Source: three-view drawing plus pictorial views. Frame: mm from the lowest corner of the part. A direction names the side the tool comes from. Coordinates: 2 decimals unless noted, no trailing zeros. Order: outer loops, then holes, each group sorted by start corner. A loop starts at its lowest first (then second) coordinate and runs counter-clockwise, first axis right, second up. Notation, with made-up numbers: (37, 81.5) - (67, 81.5) arc R19 cw to (67, 98.5) - close; hole circle Ø8 at (-36.75, 62.5). An arc over 180 degrees is marked (long way). One line per question, with ' | ' between items.
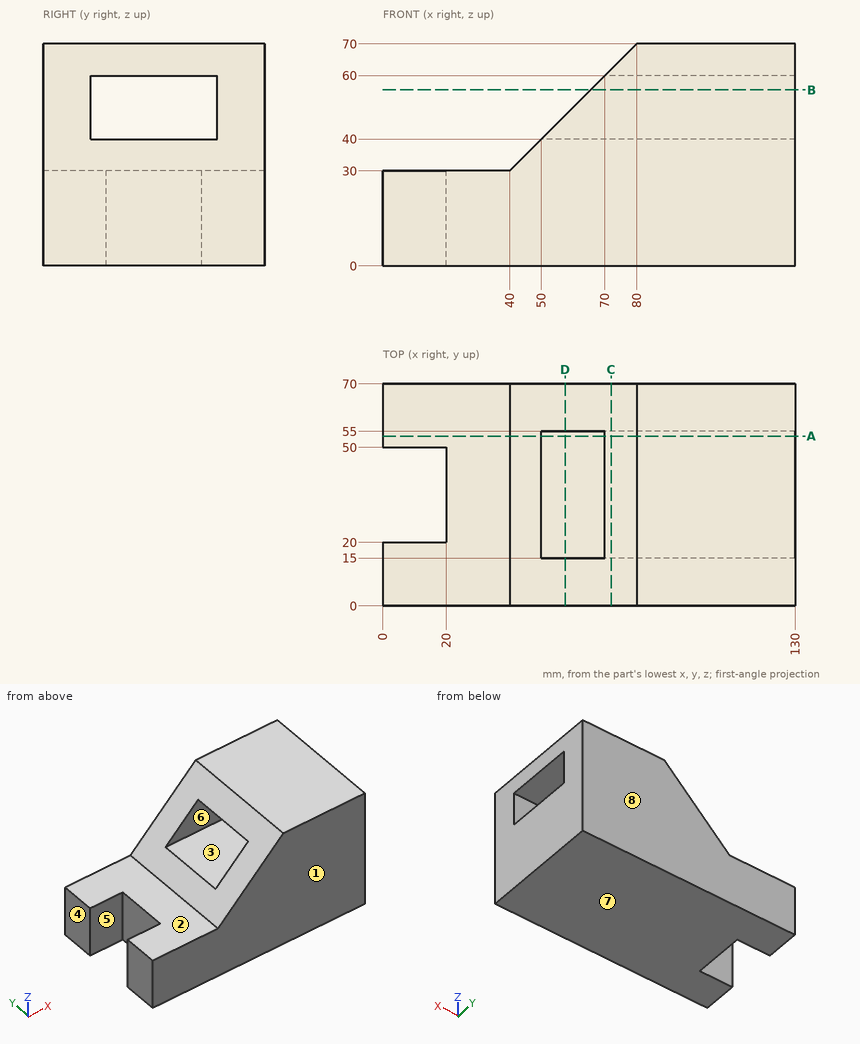
Item 1: Contact query for flat-ended pins moving along their axis: P1, Ø12, axis at y = 16.5, z = 41.5, coming from the -X side; P2, Ø4, axis at y = 12, z = 56, coming from the -X side; P3, Ø8, axis at x = 75.5, y = 40.5, coming from the +Z side. Output: stop coordinate, or through.
Data:
P1: x = 45.5 | P2: x = 64 | P3: z = 69.5
Item 2: Section B-B on z = 55.5. Return the cut outline in (x, y), and give its area (4 significant figures).
Data:
outline: (65.5, 0) - (130, 0) - (130, 15) - (65.5, 15) - close; (65.5, 55) - (130, 55) - (130, 70) - (65.5, 70) - close | area: 1,935 mm^2
Item 3: Section D-D on x = 57.5. Return the cut outline in (y, z), and give its area (4 significant figures).
Data:
outline: (0, 0) - (70, 0) - (70, 47.5) - (55, 47.5) - (55, 40) - (15, 40) - (15, 47.5) - (0, 47.5) - close | area: 3,025 mm^2
Item 4: Ray query, line 1 (Z direction, x = 118, y = 17); line 2 (Z direction, x = 27, y = 21.5); line 3 (X direction, y = 30, z = 8). Return the intervals inside material, ascending.
Data:
line 1: 0 to 40, 60 to 70 | line 2: 0 to 30 | line 3: 20 to 130
Item 5: Section C-C on x = 72. Return the cut outline in (y, z), and give its area (3 significant figures).
Data:
outline: (0, 0) - (70, 0) - (70, 62) - (0, 62) - close; hole (15, 40) - (55, 40) - (55, 60) - (15, 60) - close | area: 3,540 mm^2
Item 6: Draft query along Z for the marked faces 6, 7 and 8. Return one class per face: released by +Z, released by -Z, zero draft, split by the parting line, or undercut.
Data:
face 6: undercut | face 7: released by -Z | face 8: zero draft
Item 7: Access query for the marked faces 1, 2, 3, 4 and 5. Directions: +Z, -Z, +X, -X, +Y, -Y. A direction counts if a zero-diameter tool reaches every point of the face in a straight line with its end or side. Return the directions, or none.
Data:
face 1: +Z, -Z, +X, -X, -Y | face 2: +Z, -X, +Y, -Y | face 3: +X, -X | face 4: +Z, -Z, -X, +Y, -Y | face 5: +Z, -Z, -X
Item 8: Section A-A on y = 53.5. Return the cut outline in (x, z), and give its area (3 significant figures).
Data:
outline: (0, 0) - (130, 0) - (130, 40) - (50, 40) - (40, 30) - (0, 30) - close; (70, 60) - (130, 60) - (130, 70) - (80, 70) - close | area: 5,300 mm^2
